The model under review builds one solid part; all positions refer to its coordinate system, in mm. Face numbers are marked on the shaded views. A direction names the side the tool comes from. Round coordinates to 2 decimals unless told otherwise and drop trailing zeros. Loops run counter-clockwise (first coordinate to the right, second up) from the corner with the lowest first, then second, coordinate; pieces in that order, holes last. Notation, with made-up numbers: (30, 44.25) -> (34, 44.25) arc R27 cw to (34, 79.25) -> close; hole circle Ø8 at (82, 75). An arc over 180 degrees is marked (long way). Use CSV: the item, a comma, the result in double quotes. Start each with the question number.
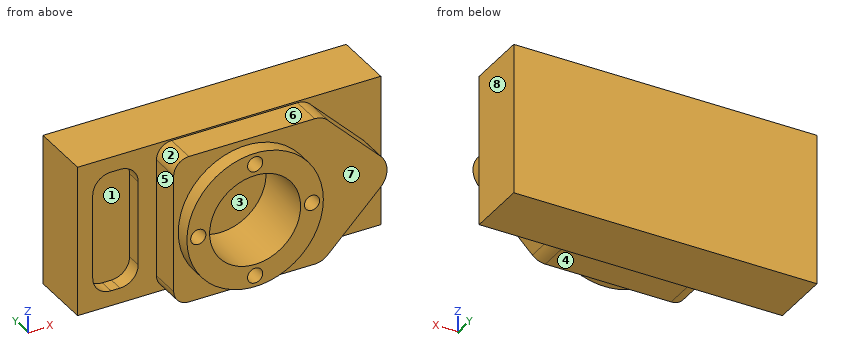
```python
from build123d import *

# Parameters (mm, degrees)
F0_W     = 200
F0_H     = 100
F1_DEPTH = 40
F2_R     = 30
F3_DEPTH = 10
F4_R     = 30
F5_DEPTH = 20
F6_R     = 45
F6_R_2   = 30
F7_DEPTH = 10
F8_R     = 5
F9_DEPTH = 25


with BuildPart() as f1:
    # F0 (on Front) → F1 (new body)
    with BuildSketch(Plane.XZ):
        with Locations((-100, 50)):
            Rectangle(F0_W, F0_H)
    extrude(amount=F1_DEPTH)

    # F2 (on face) → F3 (cut)
    with BuildSketch(Plane.XZ.offset(40)):
        with BuildLine():
            Line((-172, 90), (-178, 90))
            ThreePointArc((-178, 90), (-186.4852813742, 86.4852813742), (-190, 78))
            Line((-190, 78), (-190, 22))
            ThreePointArc((-190, 22), (-186.4852813742, 13.5147186258), (-178, 10))
            Line((-178, 10), (-172, 10))
            ThreePointArc((-172, 10), (-163.5147186258, 13.5147186258), (-160, 22))
            Line((-160, 22), (-160, 78))
            ThreePointArc((-160, 78), (-163.5147186258, 86.4852813742), (-172, 90))
        make_face()
        with Locations((-100, 50)):
            Circle(F2_R)
    extrude(amount=-F3_DEPTH, mode=Mode.SUBTRACT)

    # F4 (on face) → F5 (join)
    with BuildSketch(Plane.XZ.offset(40)):
        with BuildLine():
            ThreePointArc((-138, 99), (-145.0710678119, 96.0710678119), (-148, 89))
            Line((-148, 89), (-148, 11))
            ThreePointArc((-148, 11), (-145.0710678119, 3.9289321881), (-138, 1))
            Line((-138, 1), (-54.98, 1))
            ThreePointArc((-54.98, 1), (-50.3814469261, 1.9160787793), (-46.485, 4.5244483955))
            Line((-46.485, 4.5244483955), (-11.6992693535, 39.39))
            ThreePointArc((-11.6992693535, 39.39), (-7.3180325381, 50.004327625), (-11.7274004602, 60.607))
            Line((-11.7274004602, 60.607), (-45.6005130737, 94.485))
            ThreePointArc((-45.6005130737, 94.485), (-49.7751945281, 97.8124927746), (-54.98, 99))
            Line((-54.98, 99), (-138, 99))
        make_face()
        with Locations((-100, 50)):
            Circle(F4_R, mode=Mode.SUBTRACT)
    extrude(amount=F5_DEPTH)

    # F6 (on face) → F7 (join)
    with BuildSketch(Plane.XZ.offset(60)):
        with Locations((-100, 50)):
            Circle(F6_R)
        with Locations((-100, 50)):
            Circle(F6_R_2, mode=Mode.SUBTRACT)
    extrude(amount=F7_DEPTH)

    # F8 (on face) → F9 (cut)
    with BuildSketch(Plane.XZ.offset(70)):
        with Locations((-100, 87.5)):
            Circle(F8_R)
        with Locations((-137.5, 50)):
            Circle(F8_R)
        with Locations((-100, 12.5)):
            Circle(F8_R)
        with Locations((-62.5, 50)):
            Circle(F8_R)
    extrude(amount=-F9_DEPTH, mode=Mode.SUBTRACT)


solid = f1.part
```
1. Take a section at C-C, the plane x = -83.5. Give the boundary of the cut face in (y, z), then the cut area to 3 significant figures.
2. For the marked faces 5, 6, 7 and 8, list the 3-axis set-ups (+Z, -Z, +X, -X, +Y, -Y) from which the entire face can be reached by the end or side of a thin tool; tool diameter is ignored.
3. Take a section at D-D, the plane x = -151. Give the boundary of the cut face in (y, z), then the cut area to 3 significant figures.
4. Take a section at A-A, the plane y = -35. Give the boundary of the cut face in (x, z).
5. Clearance check with flat-ended pins moving along their axes: P1, Ø10, axis at y = -53.5, z = 35, coming from the -X side; P2, Ø1, axis at x = -82, y = -43, coming from the +Z side; P3, Ø22, axis at x = -88.5, y = -49, coming from the +Z side; P4, Ø2, axis at x = -43, y = -55.5, coming from the +Z side. State where each tip first meets the part, or that it passes through.
6. Take a section at B-B, the plane x = -32. Give the boundary of the cut face in (y, z), then the cut area to 3 significant figures.
7. For line 1 along Z through (x, y) = (-100, -51); line 2 along Z through (x, y) = (-100, -61); line 3 along Z through (x, y) = (-175, -38.5), list the stretches that pass through material, from the lowest coordinate up. Write a range as from..to.
8. The part is to be moulded in two halves that separate along X. For the marked faces 1, 2, 3 and 4, say which applies: pulls with the +X half, pulls with the -X half, needs draft (parallel to the pull), parting line crosses it, or undercut.
Results:
1,outline,"(-70, 8.13) -> (-60, 8.13) -> (-60, 1) -> (-40, 1) -> (-40, 0) -> (0, 0) -> (0, 100) -> (-40, 100) -> (-40, 99) -> (-60, 99) -> (-60, 91.87) -> (-70, 91.87) -> (-70, 75.05) -> (-30, 75.05) -> (-30, 24.95) -> (-70, 24.95) -> close"
1,area,"4,790 mm²"
2,face 5,"+Z, -Z, -X, -Y"
2,face 6,"+Z, +X, -X, -Y"
2,face 7,"-Y"
2,face 8,"+Z, -Z, +X, +Y, -Y"
3,outline,"(-40, 0) -> (0, 0) -> (0, 100) -> (-40, 100) -> close"
3,area,"4,000 mm²"
4,outline,"(-200, 0) -> (0, 0) -> (0, 100) -> (-200, 100) -> close; hole (-190, 22) arc R12 ccw to (-178, 10) -> (-172, 10) arc R12 ccw to (-160, 22) -> (-160, 78) arc R12 ccw to (-172, 90) -> (-178, 90) arc R12 ccw to (-190, 78) -> close; hole circle Ø60 at (-100, 50)"
5,P1,"x = -148"
5,P2,"z = 99"
5,P3,"z = 100"
5,P4,"z = 92.88"
6,outline,"(-60, 19.04) -> (-40, 19.04) -> (-40, 0) -> (0, 0) -> (0, 100) -> (-40, 100) -> (-40, 80.88) -> (-60, 80.88) -> close"
6,area,"5,240 mm²"
7,line 1,"1..7.5, 17.5..20, 80..82.5, 92.5..99"
7,line 2,"5..7.5, 17.5..20, 80..82.5, 92.5..95"
7,line 3,"0..10, 90..100"
8,face 1,"undercut"
8,face 2,"pulls with the -X half"
8,face 3,"undercut"
8,face 4,"needs draft"
